Job drawing, mm, ordinate dimensions from the low corner. One solid piece. Give positions to 0.01 mm unless a question says otherwise; leave off trailing zeros. Write each loop counter-clockwise with the first axis right and the second up, starting at its lowest first coordinate (ties: lowest second). Pieces come first, ordered by that corner, then holes. Notation, with made-up numbers: (88.25, 1) -> (111.25, 1) arc R24 cw to (111.25, 26) -> close; hole circle Ø7 at (46.5, 54). An arc over 180 degrees is marked (long way). One line per question, with ' | ' between items. Start each with the question number.
(1) Drill centre lines: probe 1 along X at (y, z) = (1.75, 40); probe 2 along Z at (x, y) = (24, 0.45); probe 3 along X at (y, z) = (2.25, 47) (1 decimal). Where is each one in solid material? Low to high. Write a range as from..to.
(2) Pin check, flat tips, straight feed: P1, Ø1.5, axis at y = 1.5, z = 47.5, coming from the +X side (1 decimal); P2, Ø0.8, axis at x = 24.5, y = 1, coming from the -Z side; P3, Ø1.5, axis at x = 2, y = 2, coming from the -Z side (1 decimal). Stop position of each tip, or through.
(3) Band-saw the part on A-A, the plane x = 40. Give the cut face in (y, z).
(4) Band-saw the part on D-D, the plane x = 24.5. Give the cut face in (y, z).
(5) Band-saw the part on B-B, the plane z = 37.5. Give the cut face in (x, y).
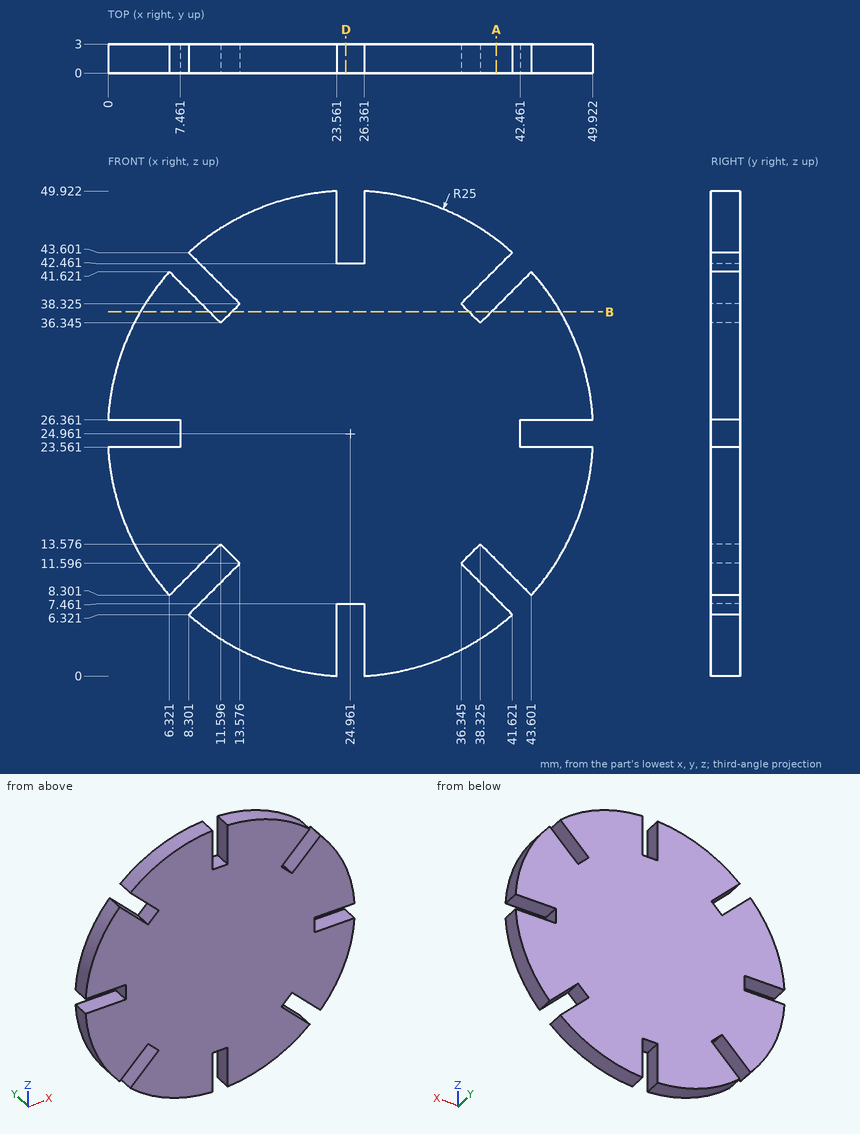
Results:
1) probe 1: x = 4.99..7.94, 11.9..38.02, 41.98..44.93 | probe 2: z = 7.46..42.46 | probe 3: x = 13.2..23.6, 26.4..36.8
2) P1: stops at x = 37.2 | P2: stops at z = 7.46 | P3: stops at z = 13.5
3) outline: (0, 4.99) -> (3, 4.99) -> (3, 7.94) -> (0, 7.94) -> close; (0, 11.9) -> (3, 11.9) -> (3, 38.02) -> (0, 38.02) -> close; (0, 41.98) -> (3, 41.98) -> (3, 44.93) -> (0, 44.93) -> close
4) outline: (0, 7.46) -> (3, 7.46) -> (3, 42.46) -> (0, 42.46) -> close
5) outline: (3.33, 0) -> (10.44, 0) -> (10.44, 3) -> (3.33, 3) -> close; (12.75, 0) -> (37.17, 0) -> (37.17, 3) -> (12.75, 3) -> close; (39.48, 0) -> (46.59, 0) -> (46.59, 3) -> (39.48, 3) -> close
